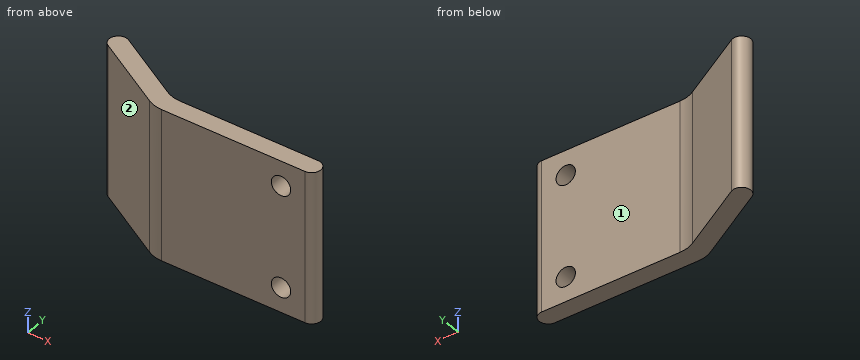
from build123d import *

# Parameters (mm, degrees)
BOSS_EXTRUDE1_DEPTH = 12.5
SKETCH2_R           = 1.6
CUT_EXTRUDE1_DEPTH  = 42.356294342
FILLET1_R           = 5


with BuildPart() as part:
    # Sketch1 → Boss-Extrude1 (new, symmetric)
    with BuildSketch(Plane.XY):
        with BuildLine():
            Line((0, 0), (-25, 0))
            Line((-25, 0), (-37.990381057, 7.5))
            ThreePointArc((-37.990381057, 7.5), (-38.539419162, 9.549038106), (-36.490381057, 10.098076211))
            Line((-36.490381057, 10.098076211), (-24.196152423, 3))
            Line((-24.196152423, 3), (0, 3))
            ThreePointArc((0, 3), (1.5, 1.5), (0, 0))
        make_face()
    extrude(amount=BOSS_EXTRUDE1_DEPTH, both=True)

    # Sketch2 → Cut-Extrude1 (cut, symmetric)
    with BuildSketch(Plane(origin=(0, 3, 0), x_dir=(1, 0, 0), z_dir=(0, 1, 0))):
        with Locations(Location((-3.968168997, -8.4, 0), (0, 0, 270))):
            Circle(SKETCH2_R)
    cut_extrude1 = extrude(amount=CUT_EXTRUDE1_DEPTH, both=True, mode=Mode.SUBTRACT)

    # Mirror1: Cut-Extrude1 across plane
    add(cut_extrude1.mirror(Plane.XY), mode=Mode.SUBTRACT)

    # Fillet1
    fillet1_edges = [part.edges().sort_by_distance(p)[0] for p in [
        (-25, 0, 0),
        (-24.196152423, 3, 0),
    ]]
    fillet(fillet1_edges, radius=FILLET1_R)


solid = part.part
Geometry check sheet. Reference: the model listing, model coordinates, mm. Face numbers are marked on the shaded views. A direction names the side the tool comes from. Coordinates: 2 decimals unless noted, no trailing zeros. Order: outer loops, then holes, each group sorted by start corner. A loop starts at its lowest first (then second) coordinate and runs counter-clockwise, first axis right, second up. Notation, with made-up numbers: (-33, 88) - (17, 88) arc R4 cw to (17, 95) - close; hole circle Ø1 at (38, -27.5). An arc over 180 degrees is marked (long way). Answer in a Markdown table with one row per item. Add a question column.
1) Cross-section at D-D, the plane x = -21.5. Record the cut outline in (y, z).
2) Cross-section at A-A, the plane z = 8.4. Record the cut outline in (x, y), then the cut area to 3 significant figures.
3) Cross-section at C-C, the plane y = 2. Record the cut outline in (x, z).
4) Material ranges on line 1 along X through (y, z) = (1.4, -8.4); line 2 along Y through (x, z) = (-3.5, -3.25); line 3 along X through (y, z) = (1.05, 8.4), recorded low to high. Write a range as [from, to].
5) Gauge pin test, flat ends, axial feed: P1, Ø6, axis at y = 8, z = 1, coming from the +X side; P2, Ø1.5, axis at y = 7.5, z = -1, coming from the +X side; P3, Ø1, axis at x = -18, z = -0.5, coming from the +Y side. Record the tip position at first contact, or that the pin passes through.
6) Set-up check for the marked faces 1 and 2: record each of +Z, -Z, +X, -X, +Y, -Y from which the full face is reachable in a straight line by a thin tool's end or side.
7) Cross-section at B-B, the plane z = -2. Record the cut outline in (x, y).
Check result:
| question | item | result |
|---|---|---|
| 1 | outline | (0, -12.5) - (3, -12.5) - (3, 12.5) - (0, 12.5) - close |
| 2 | outline | (-37.99, 7.5) - (-26.16, 0.67) arc R5 ccw to (-23.66, 0) - (-5.57, 0) - (-5.57, 3) - (-22.86, 3) arc R5 cw to (-25.36, 3.67) - (-36.49, 10.1) arc R1.5 ccw to start; (-2.37, 0) - (0, 0) arc R1.5 ccw to (0, 3) - (-2.37, 3) - close |
| 2 | area | 115 mm² |
| 3 | outline | (-28.46, -12.5) - (1.41, -12.5) - (1.41, 12.5) - (-28.46, 12.5) - close; hole circle Ø3.2 at (-3.97, -8.4); hole circle Ø3.2 at (-3.97, 8.4) |
| 4 | line 1 | x = [-27.42, -5.57], [-2.37, 1.5] |
| 4 | line 2 | y = [0, 3] |
| 4 | line 3 | x = [-26.82, -5.57], [-2.37, 1.43] |
| 5 | P1 | stops at x = -27.66 |
| 5 | P2 | stops at x = -30.69 |
| 5 | P3 | stops at y = 3 |
| 6 | face 1 | +Z, -Z, +X, +Y |
| 6 | face 2 | +Z, -Z, -X, -Y |
| 7 | outline | (-37.99, 7.5) - (-26.16, 0.67) arc R5 ccw to (-23.66, 0) - (0, 0) arc R1.5 ccw to (0, 3) - (-22.86, 3) arc R5 cw to (-25.36, 3.67) - (-36.49, 10.1) arc R1.5 ccw to start |
